from build123d import *

# Parameters (mm, degrees)
SM_BASE_FLANGE_1_DEPTH = 198.3
FILLET_1_R             = 3
SKETCH_6_R             = 1.65
CUT_EXTRUDE_1_DEPTH    = 299.389242433
CUT_EXTRUDE_2_REACH    = 482.769
SKETCH_7_R             = 1.65
CHAMFER_2_SIZE         = 1.6


# Sheet-metal steps are written as plain solids
with BuildPart() as part:
    # Sketch 1 → Базовая кромка1 (new body)
    with BuildSketch(Plane.XY):
        with BuildLine():
            Line((-217.2, -21.1), (-217.2, 19.3))
            ThreePointArc((-217.2, 19.3), (-216.760660172, 20.360660172), (-215.7, 20.8))
            Line((-215.7, 20.8), (215.7, 20.8))
            ThreePointArc((215.7, 20.8), (216.760660172, 20.360660172), (217.2, 19.3))
            Line((217.2, 19.3), (217.2, -21.1))
            Line((217.2, -21.1), (218.7, -21.1))
            Line((218.7, -21.1), (218.7, 19.3))
            ThreePointArc((218.7, 19.3), (217.821320344, 21.421320344), (215.7, 22.3))
            Line((215.7, 22.3), (-215.7, 22.3))
            ThreePointArc((-215.7, 22.3), (-217.821320344, 21.421320344), (-218.7, 19.3))
            Line((-218.7, 19.3), (-218.7, -21.1))
            Line((-218.7, -21.1), (-217.2, -21.1))
        make_face()
    extrude(amount=SM_BASE_FLANGE_1_DEPTH)

    # Скругление1
    fillet_1_edges = [part.edges().sort_by_distance(p)[0] for p in [
        (-217.95, -21.1, 0),
        (217.95, -21.1, 0),
        (-217.95, -21.1, 198.3),
        (217.95, -21.1, 198.3),
    ]]
    fillet(fillet_1_edges, radius=FILLET_1_R)

    # Эскиз6 → Вырез-Вытянуть1 (cut, through all)
    with BuildSketch(Plane(origin=(0, 22.3, 0), x_dir=(1, 0, 0), z_dir=(0, 1, 0))):
        with Locations(Location((-150, -5, 0), (0, 0, 270))):
            Circle(SKETCH_6_R)
        with Locations(Location((150, -5, 0), (0, 0, 270))):
            Circle(SKETCH_6_R)
    cut_extrude_1 = extrude(amount=-CUT_EXTRUDE_1_DEPTH, mode=Mode.SUBTRACT)

    # Зеркальное отражение1: Вырез-Вытянуть1 across plane
    add(cut_extrude_1.mirror(Plane(origin=(0, 0, 99.15), x_dir=(1, 0, 0), z_dir=(0, 0, -1))), mode=Mode.SUBTRACT)

    # Вырез-Вытянуть2: up to this face of the body (flat: up to its plane)
    cut_extrude_2_end = Plane(part.part.faces().sort_by_distance((-218.7, -0.890578691, 99.15))[0])
    # Эскиз7 → Вырез-Вытянуть2 (cut, up to the picked face)
    with BuildSketch(Plane(origin=(218.7, 0, 0), x_dir=(0, 0, -1), z_dir=(1, 0, 0)), mode=Mode.PRIVATE) as cut_extrude_2_sk1:
        with Locations(Location((-154.15, -13.6, 0), (0, 0, 90))):
            Circle(SKETCH_7_R)
    cut_extrude_2_tool1 = split(extrude(cut_extrude_2_sk1.sketch, amount=-CUT_EXTRUDE_2_REACH, mode=Mode.PRIVATE), bisect_by=cut_extrude_2_end, keep=Keep.BOTH, mode=Mode.PRIVATE)
    # Эскиз7 → Вырез-Вытянуть2 (cut, up to the picked face)
    with BuildSketch(Plane(origin=(218.7, 0, 0), x_dir=(0, 0, -1), z_dir=(1, 0, 0)), mode=Mode.PRIVATE) as cut_extrude_2_sk2:
        with Locations(Location((-44.15, -13.6, 0), (0, 0, 90))):
            Circle(SKETCH_7_R)
    cut_extrude_2_tool2 = split(extrude(cut_extrude_2_sk2.sketch, amount=-CUT_EXTRUDE_2_REACH, mode=Mode.PRIVATE), bisect_by=cut_extrude_2_end, keep=Keep.BOTH, mode=Mode.PRIVATE)
    add(cut_extrude_2_tool1.solids().sort_by(Axis((218.7, -13.6, 154.15), (-1, 0, 0)))[0], mode=Mode.SUBTRACT)
    add(cut_extrude_2_tool2.solids().sort_by(Axis((218.7, -13.6, 44.15), (-1, 0, 0)))[0], mode=Mode.SUBTRACT)

    # Фаска2
    # the kernel refuses this chamfer: 1.6 mm, written as the material it takes off along each edge
    with BuildSketch(Plane(origin=(-218.7, -13.6, 44.15), x_dir=(0, 1, 0), z_dir=(0, 0, -1))) as chamfer_2_piece_1:
        Polygon((1.65 + CHAMFER_2_SIZE, 0), (1.65, CHAMFER_2_SIZE), (1.65, 0), align=None)
    revolve(axis=Axis((-218.7, -13.6, 44.15), (1, 0, 0)), mode=Mode.SUBTRACT)
    with BuildSketch(Plane(origin=(-218.7, -13.6, 154.15), x_dir=(0, 1, 0), z_dir=(0, 0, -1))) as chamfer_2_piece_2:
        Polygon((1.65 + CHAMFER_2_SIZE, 0), (1.65, CHAMFER_2_SIZE), (1.65, 0), align=None)
    revolve(axis=Axis((-218.7, -13.6, 154.15), (1, 0, 0)), mode=Mode.SUBTRACT)
    with BuildSketch(Plane(origin=(-150, 22.3, 193.3), x_dir=(0, 0, -1), z_dir=(-1, 0, 0))) as chamfer_2_piece_3:
        Polygon((1.65 + CHAMFER_2_SIZE, 0), (1.65, CHAMFER_2_SIZE), (1.65, 0), align=None)
    revolve(axis=Axis((-150, 22.3, 193.3), (0, -1, 0)), mode=Mode.SUBTRACT)
    with BuildSketch(Plane(origin=(-150, 22.3, 5), x_dir=(0, 0, 1), z_dir=(-1, 0, 0))) as chamfer_2_piece_4:
        Polygon((1.65 + CHAMFER_2_SIZE, 0), (1.65, -CHAMFER_2_SIZE), (1.65, 0), align=None)
    revolve(axis=Axis((-150, 22.3, 5), (0, 1, 0)), mode=Mode.SUBTRACT)
    with BuildSketch(Plane(origin=(150, 22.3, 5), x_dir=(0, 0, 1), z_dir=(-1, 0, 0))) as chamfer_2_piece_5:
        Polygon((1.65 + CHAMFER_2_SIZE, 0), (1.65, -CHAMFER_2_SIZE), (1.65, 0), align=None)
    revolve(axis=Axis((150, 22.3, 5), (0, 1, 0)), mode=Mode.SUBTRACT)
    with BuildSketch(Plane(origin=(218.7, -13.6, 44.15), x_dir=(0, 1, 0), z_dir=(0, 0, -1))) as chamfer_2_piece_6:
        Polygon((1.65 + CHAMFER_2_SIZE, 0), (1.65, -CHAMFER_2_SIZE), (1.65, 0), align=None)
    revolve(axis=Axis((218.7, -13.6, 44.15), (1, 0, 0)), mode=Mode.SUBTRACT)
    with BuildSketch(Plane(origin=(218.7, -13.6, 154.15), x_dir=(0, 1, 0), z_dir=(0, 0, -1))) as chamfer_2_piece_7:
        Polygon((1.65 + CHAMFER_2_SIZE, 0), (1.65, -CHAMFER_2_SIZE), (1.65, 0), align=None)
    revolve(axis=Axis((218.7, -13.6, 154.15), (1, 0, 0)), mode=Mode.SUBTRACT)
    with BuildSketch(Plane(origin=(150, 22.3, 193.3), x_dir=(0, 0, -1), z_dir=(-1, 0, 0))) as chamfer_2_piece_8:
        Polygon((1.65 + CHAMFER_2_SIZE, 0), (1.65, CHAMFER_2_SIZE), (1.65, 0), align=None)
    revolve(axis=Axis((150, 22.3, 193.3), (0, -1, 0)), mode=Mode.SUBTRACT)


solid = part.part
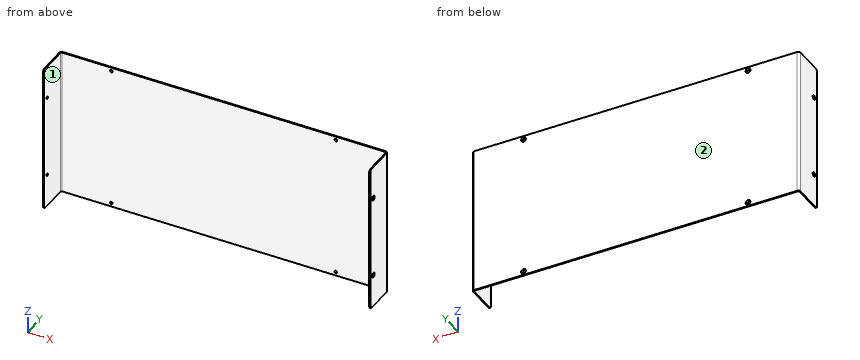
Source: CAD feature listing. Evaluate the final solid. Frame: model axes, mm. Face numbers are marked on the shaded views. A direction names the side the tool comes from. Round coordinates to 2 decimals unless told otherwise and drop trailing zeros. Order: outer loops, then holes, each group sorted by start corner. A loop starts at its lowest first (then second) coordinate and runs counter-clockwise, first axis right, second up. Notation, with made-up numbers: (52, 87.5) - (65, 87.5) arc R13 ccw to (65, 106.5) - close; hole circle Ø1 at (-2.5, -31). An arc over 180 degrees is marked (long way). Use a Markdown table: item, result. Add a question column.
1. Section query A-A (y = 15). Return the cut outline in (x, z).
2. First-contact query: pin 1 (2 mm diameter, centred on x = 100, z = 128.5, fed in from -Y). Flat tip, straight axial feed; report the tip coordinate or a pass-through.
3. Set-up query: the marked faces 1 and 2. Return all of +Z, -Z, +X, -X, +Y, -Y with unobstructed straight access to the full face (end or side cutting, diameter ignored); none if empty.
4. Section query B-B (z = 20). Return the cut outline in (x, y).
5. Section query C-C (x = 2.5). Return the cut outline in (y, z).
6. Line query: probe 1 along X at (y, z) = (14.5, 35); probe 2 along Y at (x, z) = (-125.5, 45.5); probe 3 along X at (y, z) = (20.5, 152). Output: solid intervals per line, ascending.
Derived:
| question | item | result |
|---|---|---|
| 1 | outline | (-218.7, 0) - (-217.2, 0) - (-217.2, 198.3) - (-218.7, 198.3) - close; (217.2, 0) - (218.7, 0) - (218.7, 198.3) - (217.2, 198.3) - close |
| 2 | pin 1 | y = 20.8 |
| 3 | face 1 | +Z, -Z, -Y |
| 3 | face 2 | +Z, -Z, +X, -X, +Y |
| 4 | outline | (-218.7, -21.1) - (-217.2, -21.1) - (-217.2, 19.3) arc R1.5 cw to (-215.7, 20.8) - (215.7, 20.8) arc R1.5 cw to (217.2, 19.3) - (217.2, -21.1) - (218.7, -21.1) - (218.7, 19.3) arc R3 ccw to (215.7, 22.3) - (-215.7, 22.3) arc R3 ccw to (-218.7, 19.3) - close |
| 5 | outline | (20.8, 0) - (22.3, 0) - (22.3, 198.3) - (20.8, 198.3) - close |
| 6 | probe 1 | -218.7 to -217.2, 217.2 to 218.7 |
| 6 | probe 2 | 20.8 to 22.3 |
| 6 | probe 3 | -218.45 to -216.6, 216.6 to 218.45 |
